Design review of the part built by this model. Coordinates are the model's own, in mm. Face numbers are marked on the shaded views. A direction names the side the tool comes from. Coordinates: 2 decimals unless noted, no trailing zeros. Loops run counter-clockwise (first coordinate to the right, second up) from the corner with the lowest first, then second, coordinate; pieces in that order, holes last. Notation, with made-up numbers: (-26, 8.25) - (7, 8.25) arc R11 ccw to (7, 28.25) - close; hole circle Ø10 at (-27, 73.5). An arc over 180 degrees is marked (long way). Use one line per item in the form item = value. Start each with the question number.
(1) Add section B-B (y = 15.25). State the section outline as (x, z) points (3 decimals).
(2) Tool access review of the marked faces 1 and 2: name each direction out of +Z, -Z, +X, -X, +Y, -Y from which nothing blocks a thin tool from reaching the whole face with its end or side.
(3) Add section A-A (z = 91). State the section outline as (x, y) points (3 decimals).
(4) Clearance check with flat-ended pins moving along their axes: pin 1 Ø3 at (x, z) = (12.7, 20) entering from -Y; pin 2 Ø8 at (y, z) = (11, 119.5) entering from -X (3 decimals); pin 3 Ø1.5 at (x, z) = (18.5, 258) entering from +Y (3 decimals). State where each tip first meets the part, or that it passes through.
(5) Add section C-C (x = 6). State the section outline as (y, z) points (3 decimals).
(6) For L1, parallel to X at y = 0.65, z = 20; L2, parallel to Y at x = 10.5, z = 67 (3 decimals); L3, parallel to X at y = 8, z = 153.5 (3 decimals), list the stretches that pass through material, from the lowest coordinate up.
```python
from build123d import *

# Parameters (mm, degrees)
BOSS_EXTRUDE1_DEPTH = 310
SKETCH2_R           = 2
CUT_EXTRUDE1_DEPTH  = 310


with BuildPart() as part:
    # Sketch1 → Boss-Extrude1 (new body)
    with BuildSketch(Plane.XY):
        Polygon((0, 0), (25.4, 0), (25.4, 25.4), (22.225, 25.4), (22.225, 3.175), (0, 3.175), align=None)
    extrude(amount=BOSS_EXTRUDE1_DEPTH)

    # Sketch2 → Cut-Extrude1 (cut)
    with BuildSketch(Plane.XZ):
        with Locations(Location((12.7, 290, 0), (0, 0, 270))):
            Circle(SKETCH2_R)
        with Locations(Location((12.7, 20, 0), (0, 0, 270))):
            Circle(SKETCH2_R)
    extrude(amount=-CUT_EXTRUDE1_DEPTH, mode=Mode.SUBTRACT)


solid = part.part
```
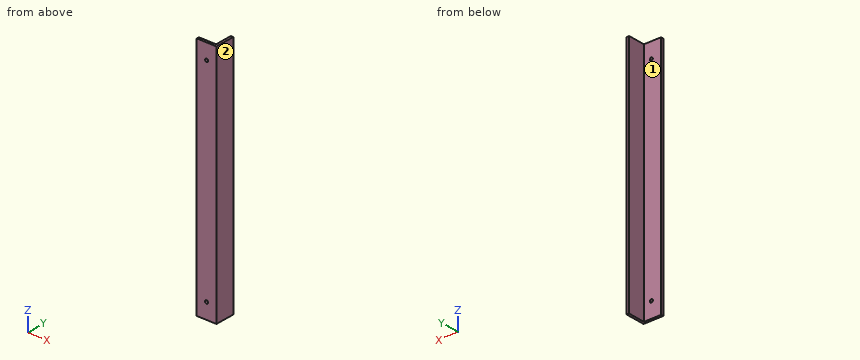
Computed values:
q1.outline = (22.225, 0) - (25.4, 0) - (25.4, 310) - (22.225, 310) - close
q2.face_1 = +Z, -Z, -X, +Y
q2.face_2 = +Z, -Z, +X, +Y, -Y
q3.outline = (0, 0) - (25.4, 0) - (25.4, 25.4) - (22.225, 25.4) - (22.225, 3.175) - (0, 3.175) - close
q4.pin_1 = through
q4.pin_2 = 22.225
q4.pin_3 = 3.175
q5.outline = (0, 0) - (3.175, 0) - (3.175, 310) - (0, 310) - close
q6.L1 = 0 to 10.7, 14.7 to 25.4
q6.L2 = 0 to 3.175
q6.L3 = 22.225 to 25.4
